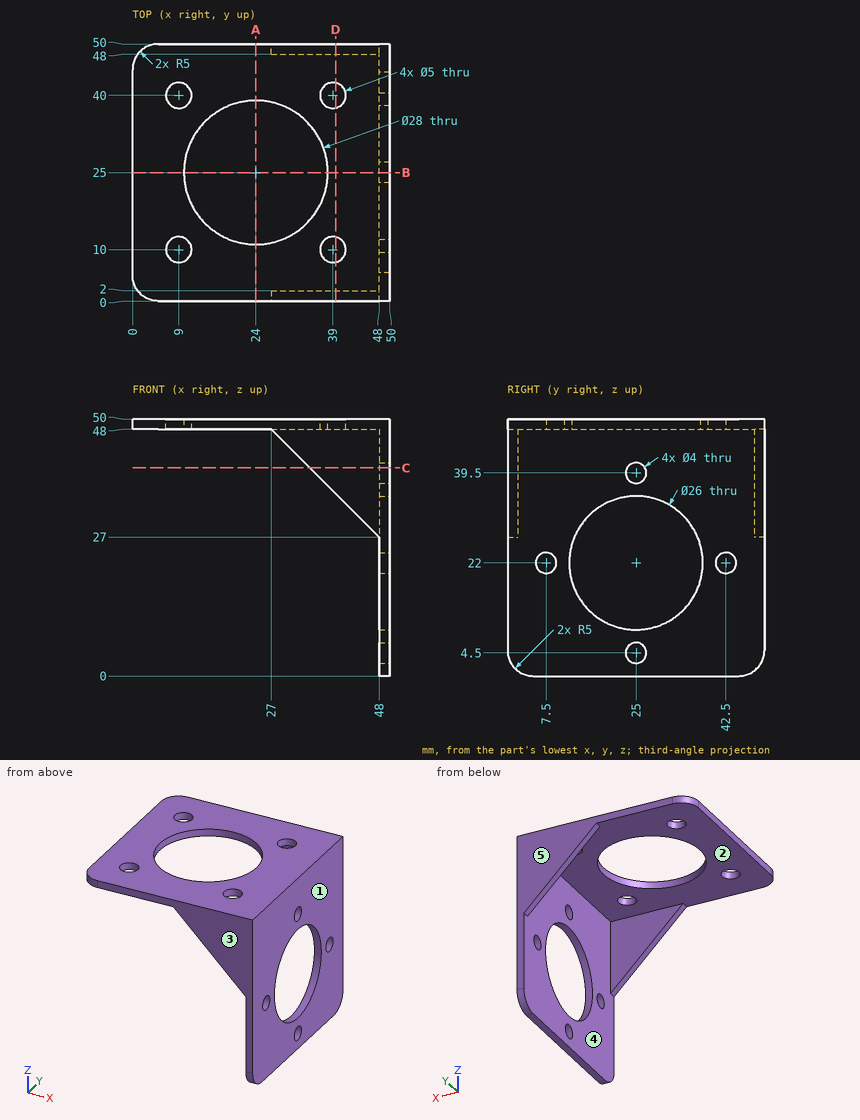
Here's the drawing with two shaded views (mm, measured from the low corner). I have some questions. A direction names the side the tool comes from. Round coordinates to 2 decimals unless told otherwise and drop trailing zeros. Loops run counter-clockwise (first coordinate to the right, second up) from the corner with the lowest first, then second, coordinate; pieces in that order, holes last.
Item 1: If we mould it in two halves opening along Y, with no side actions, what happens to the marked faces 1, 2 and 3? For each: +Y half, -Y half, draft (parallel to the pull), parting line (faces both ways), or undercut.
Item 2: Suppose I cut it at C-C, the plane z = 40.5. Write out the boundary of the cut face in (x, y).
Item 3: Will these pins go through, and if not, where does the flat tip stop? pin 1 Ø3 at (y, z) = (7.5, 22) entering from +X; pin 2 Ø5 at (y, z) = (16, 30) entering from -X; pin 3 Ø4 at (x, y) = (35, 32) entering from -Z.
Item 4: Suppose I cut it at A-A, the plane x = 24. Write out the boundary of the cut face in (y, z), then the cut area to 3 significant figures.
Item 5: Suppose I cut it at D-D, the plane x = 39.5. Write out the boundary of the cut face in (y, z).
Item 6: Please list where these lines run through material, in increasing order: L1, parallel to Z at x = 49.5, y = 42.5; L2, parallel to Y at x = 49.5, z = 39.5; L3, parallel to Z at x = 14.5, y = 7.
Item 7: Suppose I cut it at B-B, the plane y = 25. Write out the boundary of the cut face in (x, z).
Item 8: Which directions (+Z, -Z, +X, -X, +Y, -Y) give clear straight access to the entire face, cutting with the end or side of a thin tool? Please do the marked faces 4 and 5.
Reported:
1. face 1: draft
1. face 2: undercut
1. face 3: -Y half
2. outline: (34.5, 0) - (50, 0) - (50, 23.27) - (48, 23.27) - (48, 2) - (34.5, 2) - close; (34.5, 48) - (48, 48) - (48, 26.73) - (50, 26.73) - (50, 50) - (34.5, 50) - close
3. pin 1: passes through
3. pin 2: stops at x = 48
3. pin 3: stops at z = 48
4. outline: (0, 48) - (11, 48) - (11, 50) - (0, 50) - close; (39, 48) - (50, 48) - (50, 50) - (39, 50) - close
4. area: 44.0 mm2
5. outline: (0, 35.5) - (2, 35.5) - (2, 48) - (7.55, 48) - (7.55, 50) - (0, 50) - close; (12.45, 48) - (37.55, 48) - (37.55, 50) - (12.45, 50) - close; (42.45, 48) - (48, 48) - (48, 35.5) - (50, 35.5) - (50, 50) - (42.45, 50) - close
6. L1: z = 0 to 20, 24 to 50
6. L2: y = 0 to 23, 27 to 50
6. L3: z = 48 to 50
7. outline: (0, 48) - (10, 48) - (10, 50) - (0, 50) - close; (38, 48) - (48, 48) - (48, 41.5) - (50, 41.5) - (50, 50) - (38, 50) - close; (48, 0) - (50, 0) - (50, 2.5) - (48, 2.5) - close; (48, 6.5) - (50, 6.5) - (50, 9) - (48, 9) - close; (48, 35) - (50, 35) - (50, 37.5) - (48, 37.5) - close
8. face 4: -Z, -X
8. face 5: +Z, -Z, +X, -X, +Y
